The listing builds one solid part. Answer for the finished solid, in the listing's coordinates (mm). Coordinates: 2 decimals unless noted, no trailing zeros. Order: outer loops, then holes, each group sorted by start corner. A loop starts at its lowest first (then second) coordinate and runs counter-clockwise, first axis right, second up.
from build123d import *

# Parameters (mm, degrees)
SKETCH_R        = 2.1
PAD_DEPTH       = 100
CHAMFER_1_ANGLE = 45
CHAMFER_1_SIZE  = 1.25
CHAMFER_2_ANGLE = 45
CHAMFER_2_SIZE  = 1.25
CHAMFER_3_ANGLE = 45
CHAMFER_3_SIZE  = 1.25
CHAMFER_4_ANGLE = 45
CHAMFER_4_SIZE  = 1.25
CHAMFER_5_ANGLE = 45
CHAMFER_5_SIZE  = 1.25
CHAMFER_6_ANGLE = 45
CHAMFER_6_SIZE  = 1.25
CHAMFER_7_ANGLE = 45
CHAMFER_7_SIZE  = 1.25
CHAMFER_8_ANGLE = 45
CHAMFER_8_SIZE  = 1.25
FILLET_R        = 0.2


with BuildPart() as part:
    # Sketch → Pad (new body)
    with BuildSketch(Plane.XY):
        Polygon((0, 3.723883), (0.176777, 3.90066), (2.84, 3.90066), (5.49934, 6.56), (5.49934, 8.2), (3.1, 8.2), (3.1, 10), (10, 10), (10, 3.1), (8.2, 3.1), (8.2, 5.49934), (6.56, 5.49934), (3.90066, 2.84), (3.90066, 0.176777), (3.723883, 0), (3.90066, -0.176777), (3.90066, -2.84), (6.56, -5.49934), (8.2, -5.49934), (8.2, -3.1), (10, -3.1), (10, -10), (3.1, -10), (3.1, -8.2), (5.49934, -8.2), (5.49934, -6.56), (2.84, -3.90066), (0.176777, -3.90066), (0, -3.723883), (-0.176777, -3.90066), (-2.84, -3.90066), (-5.49934, -6.56), (-5.49934, -8.2), (-3.1, -8.2), (-3.1, -10), (-10, -10), (-10, -3.1), (-8.2, -3.1), (-8.2, -5.49934), (-6.56, -5.49934), (-3.90066, -2.84), (-3.90066, -0.176777), (-3.723883, 0), (-3.90066, 0.176777), (-3.90066, 2.84), (-6.56, 5.49934), (-8.2, 5.49934), (-8.2, 3.1), (-10, 3.1), (-10, 10), (-3.1, 10), (-3.1, 8.2), (-5.49934, 8.2), (-5.49934, 6.56), (-2.84, 3.90066), (-0.176777, 3.90066), align=None)
        Circle(SKETCH_R, mode=Mode.SUBTRACT)
    extrude(amount=PAD_DEPTH)

    # Chamfer 1
    chamfer_1_edges = [part.edges().sort_by_distance(p)[0] for p in [
        (-3.1, 10, 50),
    ]]
    chamfer_1_side = part.faces().sort_by_distance((-6.55, 10, 50))[0]
    chamfer(chamfer_1_edges, length=CHAMFER_1_SIZE, angle=CHAMFER_1_ANGLE, reference=chamfer_1_side)

    # Chamfer 2
    chamfer_2_edges = [part.edges().sort_by_distance(p)[0] for p in [
        (3.1, 10, 50),
    ]]
    chamfer_2_side = part.faces().sort_by_distance((3.1, 9.1, 50))[0]
    chamfer(chamfer_2_edges, length=CHAMFER_2_SIZE, angle=CHAMFER_2_ANGLE, reference=chamfer_2_side)

    # Chamfer 3
    chamfer_3_edges = [part.edges().sort_by_distance(p)[0] for p in [
        (-10, 3.1, 50),
    ]]
    chamfer_3_side = part.faces().sort_by_distance((-9.1, 3.1, 50))[0]
    chamfer(chamfer_3_edges, length=CHAMFER_3_SIZE, angle=CHAMFER_3_ANGLE, reference=chamfer_3_side)

    # Chamfer 4
    chamfer_4_edges = [part.edges().sort_by_distance(p)[0] for p in [
        (3.1, -10, 50),
    ]]
    chamfer_4_side = part.faces().sort_by_distance((6.55, -10, 50))[0]
    chamfer(chamfer_4_edges, length=CHAMFER_4_SIZE, angle=CHAMFER_4_ANGLE, reference=chamfer_4_side)

    # Chamfer 5
    chamfer_5_edges = [part.edges().sort_by_distance(p)[0] for p in [
        (-3.1, -10, 50),
    ]]
    chamfer_5_side = part.faces().sort_by_distance((-3.1, -9.1, 50))[0]
    chamfer(chamfer_5_edges, length=CHAMFER_5_SIZE, angle=CHAMFER_5_ANGLE, reference=chamfer_5_side)

    # Chamfer 6
    chamfer_6_edges = [part.edges().sort_by_distance(p)[0] for p in [
        (10, 3.1, 50),
    ]]
    chamfer_6_side = part.faces().sort_by_distance((10, 6.55, 50))[0]
    chamfer(chamfer_6_edges, length=CHAMFER_6_SIZE, angle=CHAMFER_6_ANGLE, reference=chamfer_6_side)

    # Chamfer 7
    chamfer_7_edges = [part.edges().sort_by_distance(p)[0] for p in [
        (10, -3.1, 50),
    ]]
    chamfer_7_side = part.faces().sort_by_distance((9.1, -3.1, 50))[0]
    chamfer(chamfer_7_edges, length=CHAMFER_7_SIZE, angle=CHAMFER_7_ANGLE, reference=chamfer_7_side)

    # Chamfer 8
    chamfer_8_edges = [part.edges().sort_by_distance(p)[0] for p in [
        (-10, -3.1, 50),
    ]]
    chamfer_8_side = part.faces().sort_by_distance((-10, -6.55, 50))[0]
    chamfer(chamfer_8_edges, length=CHAMFER_8_SIZE, angle=CHAMFER_8_ANGLE, reference=chamfer_8_side)

    # Fillet
    fillet_edges = [part.edges().sort_by_distance(p)[0] for p in [
        (10, 10, 50),
        (-10, 10, 50),
        (-10, -10, 50),
        (10, -10, 50),
    ]]
    fillet(fillet_edges, radius=FILLET_R)


solid = part.part
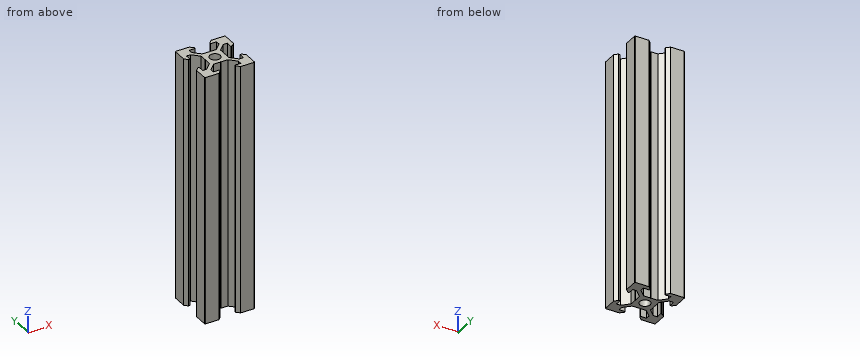
1) Each of these flat-tipped pins is pushed along its axis until it touches: P1, Ø0.8, axis at y = 2, z = 45, coming from the -X side; P2, Ø3, axis at x = -2, z = 34.5, coming from the -Y side; P3, Ø2, axis at x = 0, y = 1, coming from the -Z side; P4, Ø3, axis at y = -1.5, z = 29.5, coming from the -X side. Where does it stop, or does it pass through?
2) Section A-A (x = -1.25) is taken. Give the vertices of the cut face in (y, z).
3) Consider L1, parallel to Y at x = 0, z = 74; L2, parallel to X at y = 3.5, z = 59; L3, parallel to X at y = -8.5, z = 28. Determine where each line is inside the solid, lowest interval first.
Filled sheet:
1. P1: stops at x = -3.9
1. P2: stops at y = -9.15
1. P3: passes through
1. P4: stops at x = -4.06
2. outline: (-3.9, 0) - (-1.69, 0) - (-1.69, 100) - (-3.9, 100) - close; (1.69, 0) - (3.9, 0) - (3.9, 100) - (1.69, 100) - close
3. L1: y = -3.72 to -2.1, 2.1 to 3.72
3. L2: x = -9.15 to -8.2, -4.56 to 4.56, 8.2 to 9.15
3. L3: x = -10 to -3.1, 3.1 to 10
